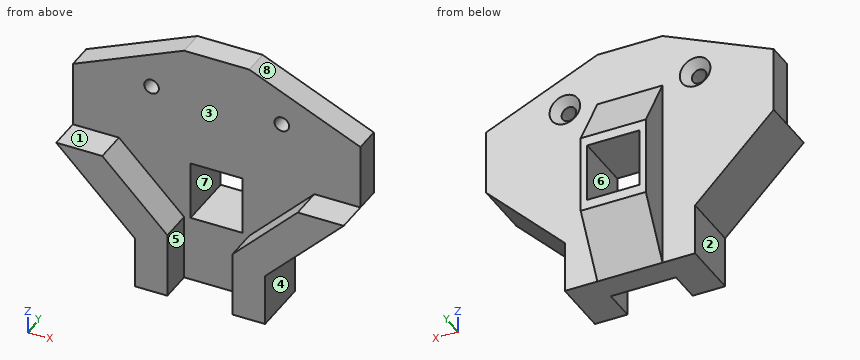
from build123d import *

# Parameters (mm, degrees)
EXTRUDE_1_DEPTH             = 10
EXTRUDE_1_2_DEPTH           = 10
EXTRUDE_2_DEPTH             = 8
HOLE_WIZARD_M41_D           = 4.5
HOLE_WIZARD_M41_CSINK_D     = 9.4
HOLE_WIZARD_M41_CSINK_ANGLE = 90
EXTRUDE_3_DEPTH             = 10
SKETCH_8_W                  = 16
SKETCH_8_H                  = 18
CUT_EXTRUDE_1_DEPTH         = 20


with BuildPart() as part:
    # Sketch 1 → Extrude 1 (new body)
    with BuildSketch(Plane(origin=(0, 0, 0), x_dir=(1, 0, 0), z_dir=(0, 1, 0))):
        Polygon((-30, 20), (-44.142135624, 20), (-20, 44.142135624), (-20, 60), (-10, 60), (-10, 40), align=None)
    extrude(amount=EXTRUDE_1_DEPTH)



with BuildPart() as body_2:
    # Sketch 1 → Extrude 1 2 (new body)
    with BuildSketch(Plane(origin=(0, 0, 0), x_dir=(1, 0, 0), z_dir=(0, 1, 0))):
        Polygon((30, 20), (10, 40), (10, 60), (20, 60), (20, 44.142135624), (44.142135624, 20), align=None)
    extrude(amount=EXTRUDE_1_2_DEPTH)


with BuildPart() as part_1:
    add(part.part)

    add(body_2.part)  # Extrude 2 merges body 2
    # Sketch 2 → Extrude 2 (add)
    with BuildSketch(Plane(origin=(0, 10, 0), x_dir=(1, 0, 0), z_dir=(0, 1, 0))):
        Polygon((44.142135624, 20), (20, 44.142135624), (20, 60), (10, 60), (-10, 60), (-20, 60), (-20, 44.142135624), (-44.142135624, 20), (-44.142135624, 0), (-10, -15), (10, -15), (44.142135624, 0), align=None)
    extrude(amount=EXTRUDE_2_DEPTH)

    # Hole Wizard M41 (through all)
    with Locations(Plane(origin=(0, 18, 0), x_dir=(1, 0, 0), z_dir=(0, 1, 0))):
        with Locations((-20, 0), (20, 0)):
            CounterSinkHole(HOLE_WIZARD_M41_D / 2, HOLE_WIZARD_M41_CSINK_D / 2, counter_sink_angle=HOLE_WIZARD_M41_CSINK_ANGLE)

    # Sketch 7 → Extrude 3 (add, symmetric)
    with BuildSketch(Plane(origin=(0, 0, 0), x_dir=(0, 0, -1), z_dir=(1, 0, 0))):
        Polygon((44.142135624, 18), (60, 18), (42.679491924, 28), (18.679491924, 28), (1.358983849, 18), align=None)
    extrude(amount=EXTRUDE_3_DEPTH, both=True)

    # Sketch 8 → Cut-Extrude 1 (cut)
    with BuildSketch(Plane(origin=(0, 28, 0), x_dir=(1, 0, 0), z_dir=(0, 1, 0))):
        with Locations((0, 30.679491924)):
            Rectangle(SKETCH_8_W, SKETCH_8_H)
    extrude(amount=-CUT_EXTRUDE_1_DEPTH, mode=Mode.SUBTRACT)


solid = part_1.part
Build history of the part. All positions in model axes, mm. Face numbers are marked on the shaded views. A direction names the side the tool comes from. Round coordinates to 2 decimals unless told otherwise and drop trailing zeros. Write each loop counter-clockwise with the first axis right and the second up, starting at its lowest first coordinate (ties: lowest second). Pieces come first, ordered by that corner, then holes. Notation, with made-up numbers: (68.25, 17.5) -> (124.25, 17.5) arc R16 ccw to (124.25, 46.5) -> close; hole circle Ø9 at (11.25, -11). An arc over 180 degrees is marked (long way). Write item = value, one per line.
(1) Probe L1, parallel to X at y = 21.75, z = -30; L2, parallel to Y at x = 15, z = -8; L3, parallel to X at y = 9.75, z = -39. List the from-to ranges inside material, lowest first.
Answer:
L1 = -10 to -8, 8 to 10
L2 = 10 to 18
L3 = -25.14 to -11, 11 to 25.14
(2) Flat gauge pins, fed straight in: pin 1 (2 mm diameter, centred on x = 2.5, z = 7.5, fed in from +Y); pin 2 (10 mm diameter, centred on x = 26, y = 8.5, fed in from -Z); pin 3 (3 mm diameter, centred on y = 5.5, z = -45, fed in from -X). Where does each tip first touch, or does it go through?
Answer:
pin_1 = 18
pin_2 = -43.14
pin_3 = -20.64
(3) Band-saw the part on C-C (z = -34.5). Give the cut face in (x, y), then the cut area to 3 significant figures.
Answer:
outline = (-29.64, 0) -> (-15.5, 0) -> (-15.5, 10) -> (-8, 10) -> (-8, 28) -> (-10, 28) -> (-10, 18) -> (-29.64, 18) -> close; (8, 10) -> (15.5, 10) -> (15.5, 0) -> (29.64, 0) -> (29.64, 18) -> (10, 18) -> (10, 28) -> (8, 28) -> close
area = 669 mm2
(4) Tool access for the marked faces 1, 2, 3 and 4: list every direction of +Z, -Z, +X, -X, +Y, -Y with a clear straight run to the whole face (end or side of a thin tool).
Answer:
face_1 = +Z, +X, -X, -Y
face_2 = -Z, -X, +Y, -Y
face_3 = +Z, -Y
face_4 = -Z, +X, +Y, -Y
(5) Two-plate mould, pull along Z, no slides. Class the marked faces 5, 6, 7 and 8: pulls with the +Z half, pulls with the -Z half, needs draft (parallel to the pull), parting line crosses it, or undercut.
Answer:
face_5 = needs draft
face_6 = undercut
face_7 = undercut
face_8 = pulls with the +Z half
(6) Band-saw the part on D-D (x = -38). Give the cut face in (y, z), then the cut area to 3 significant figures.
Answer:
outline = (0, -26.14) -> (18, -26.14) -> (18, 2.7) -> (10, 2.7) -> (10, -20) -> (0, -20) -> close
area = 292 mm2
(7) Band-saw the part on B-B (y = 21). Give the cut face in (x, z), then the cut area to 3 significant figures.
Answer:
outline = (-10, -54.8) -> (10, -54.8) -> (10, -6.56) -> (-10, -6.56) -> close; hole (-8, -39.68) -> (8, -39.68) -> (8, -21.68) -> (-8, -21.68) -> close
area = 677 mm2
(8) Band-saw the part on A-A (y = 5.5). Give the cut face in (x, z), then the cut area to 3 significant figures.
Answer:
outline = (-44.14, -20) -> (-20, -44.14) -> (-20, -60) -> (-10, -60) -> (-10, -40) -> (-30, -20) -> close; (10, -60) -> (20, -60) -> (20, -44.14) -> (44.14, -20) -> (30, -20) -> (10, -40) -> close
area = 983 mm2
